The model under review builds one solid part; all positions refer to its coordinate system, in mm. Face numbers are marked on the shaded views. A direction names the side the tool comes from. Coordinates: 2 decimals unless noted, no trailing zeros. Loops run counter-clockwise (first coordinate to the right, second up) from the corner with the lowest first, then second, coordinate; pieces in that order, holes last. Notation, with made-up numbers: (39, 78) -> (44, 78) arc R25 ccw to (44, 102) -> close; hole circle Ø6 at (77.25, 89). An arc over 180 degrees is marked (long way). One line per question, with ' | ' between items. Start each with the question number.
from build123d import *

# Parameters (mm, degrees)
F0_W     = 85
F0_H     = 90
F1_DEPTH = 102.5
F2_W     = 80
F2_H     = 85
F3_DEPTH = 10
F4_W     = 80
F4_H     = 85
F5_DEPTH = 90
F6_W     = 80
F6_H     = 80
F7_DEPTH = 25
F8_R     = 45


with BuildPart() as f1:
    # F0 (on Top) → F1 (new body)
    with BuildSketch(Plane.XY):
        with Locations((-11.937995, -3.484366)):
            Rectangle(F0_W, F0_H)
    extrude(amount=F1_DEPTH)

    # F2 (on face) → F3 (cut)
    with BuildSketch(Plane(origin=(0, 0, 0), x_dir=(1, 0, 0), z_dir=(0, 0, -1))):
        with Locations((-11.937995, 3.484366)):
            Rectangle(F2_W, F2_H)
    extrude(amount=-F3_DEPTH, mode=Mode.SUBTRACT)

    # F4 (on face) → F5 (cut)
    with BuildSketch(Plane.XY.offset(102.5)):
        with Locations((-11.937995, -3.484366)):
            Rectangle(F4_W, F4_H)
    extrude(amount=-F5_DEPTH, mode=Mode.SUBTRACT)

    # F6 (on face) → F7 (cut)
    with BuildSketch(Plane.XZ.offset(48.484366)):
        with Locations((-11.937995, 62.5)):
            Rectangle(F6_W, F6_H)
    extrude(amount=-F7_DEPTH, mode=Mode.SUBTRACT)

    # F8
    f8_edges = [f1.edges().sort_by_distance(p)[0] for p in [
        (-53.187995, -48.484366, 102.5),
        (29.312005, -48.484366, 102.5),
    ]]
    fillet(f8_edges, radius=F8_R)


solid = f1.part
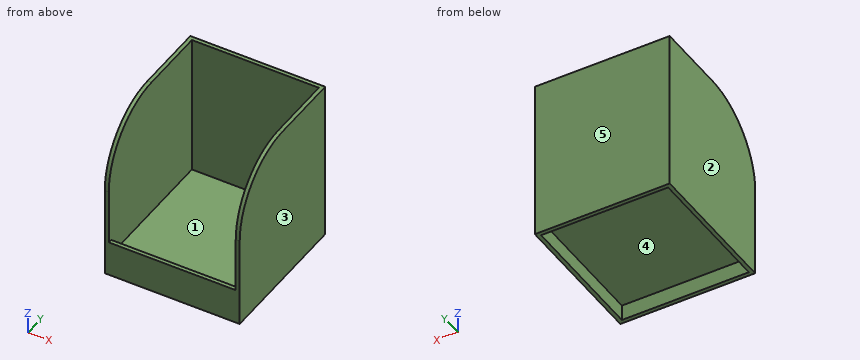
1) Machinability: for the marked faces 1 and 2, which of the approach directions +Z, -Z, +X, -X, +Y, -Y give a long, thin tool a straight path to every point of the face, cutting with its end or side? Answer none if there is none.
2) Wall thickness on L1, parallel to X at y = -23.5, z = 50; L2, parallel to Z at x = 15, y = 33.5; L3, parallel to Y at x = 5.5, z = 20.5: over which ranges is each line inside the solid? List them lowest first.
3) Consider section C-C, the plane y = 16.5. Write out the cut boundary in (x, z), plus the area to 4 significant figures.
4) Consider section A-A, the plane x = -1.5. Write out the cut boundary in (y, z).
5) Consider section B-B, the plane z = 43. Write out the cut boundary in (x, y), plus the area to 3 significant figures.
6) Insertion check: pin 1 Ø4 at (x, y) = (-21, -12) entering from -Z; pin 2 Ø2 at (x, z) = (12.5, 53.5) entering from -Y; pin 3 Ø1.2 at (x, y) = (-8, -47) entering from +Z. Each pin has a flat end and moves straight along its axis. Give the tip position at first contact, or say it passes through.
7) Consider section D-D, the plane z = 73. Write out the cut boundary in (x, y), plus the area to 3 significant figures.
8) Mouldability with a two-part tool opening along Y and no side actions: class the marked faces 3, 4 and 5 as +Y half, -Y half, draft (parallel to the pull), parting line (faces both ways), or undercut.
Filled sheet:
1) face 1: +Z | face 2: +Z, -Z, -X, +Y, -Y
2) L1: -54.44 to -51.94, 28.06 to 30.56 | L2: 10 to 12.5 | L3: -48.48 to -45.98, 39.02 to 41.52
3) outline: (-54.44, 0) -> (-51.94, 0) -> (-51.94, 10) -> (28.06, 10) -> (28.06, 0) -> (30.56, 0) -> (30.56, 102.5) -> (28.06, 102.5) -> (28.06, 12.5) -> (-51.94, 12.5) -> (-51.94, 102.5) -> (-54.44, 102.5) -> close | area: 712.5 mm^2
4) outline: (-48.48, 0) -> (-45.98, 0) -> (-45.98, 10) -> (39.02, 10) -> (39.02, 0) -> (41.52, 0) -> (41.52, 102.5) -> (39.02, 102.5) -> (39.02, 12.5) -> (-45.98, 12.5) -> (-45.98, 22.5) -> (-48.48, 22.5) -> close
5) outline: (-54.44, -48.48) -> (-51.94, -48.48) -> (-51.94, 39.02) -> (28.06, 39.02) -> (28.06, -48.48) -> (30.56, -48.48) -> (30.56, 41.52) -> (-54.44, 41.52) -> close | area: 650 mm^2
6) pin 1: z = 10 | pin 2: y = 39.02 | pin 3: z = 22.5
7) outline: (-54.44, -45.73) -> (-51.94, -45.73) -> (-51.94, 39.02) -> (28.06, 39.02) -> (28.06, -45.73) -> (30.56, -45.73) -> (30.56, 41.52) -> (-54.44, 41.52) -> close | area: 636 mm^2
8) face 3: draft | face 4: undercut | face 5: +Y half
